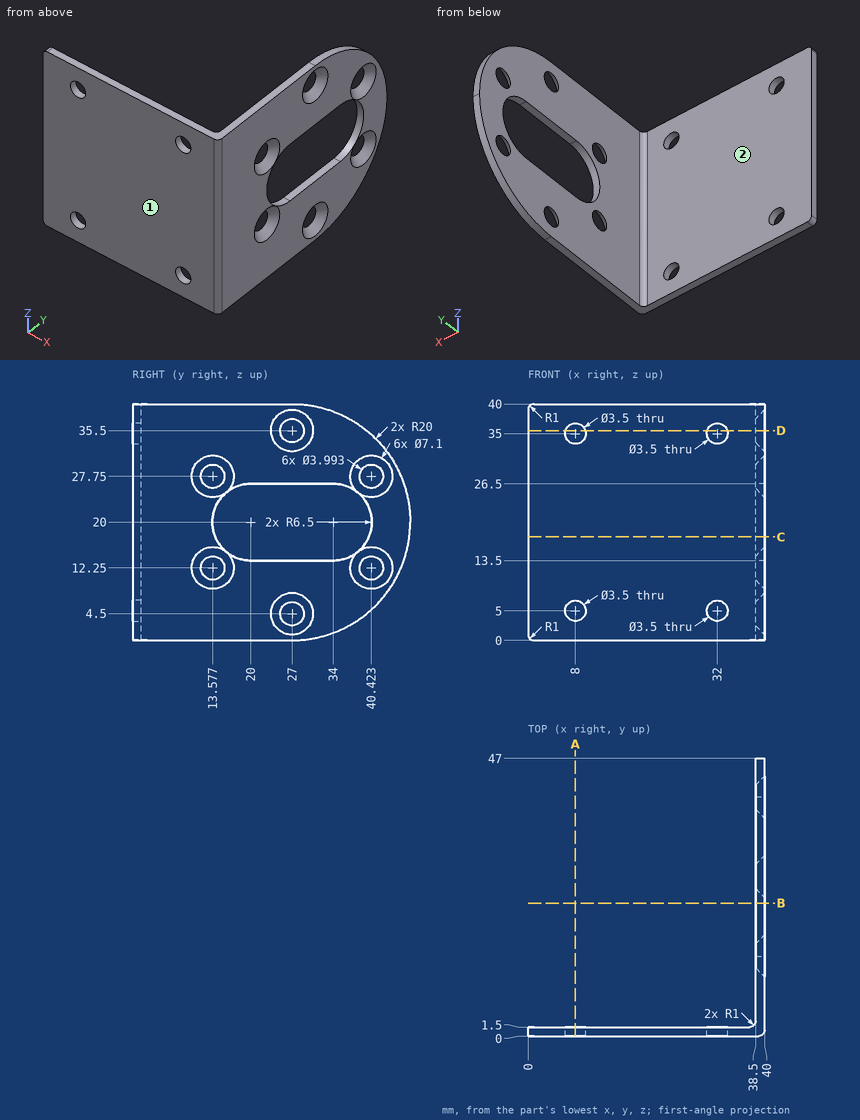
Check sheet for the drawn part. Datum: minimum x, y, z corner. Units: mm. A direction names the side the tool comes from. Give positions to 0.01 mm unless a question says otherwise; leave off trailing zeros. Write each loop counter-clockwise with the first axis right and the second up, starting at its lowest first coordinate (ties: lowest second). Pieces come first, ordered by that corner, then holes. Notation, with made-up numbers: M -31,41 L -6,41 A30 cw -6,64 Z; hole C 39,19.25 d11. An arc over 180 degrees is marked long. One line per question, with ' | ' between items.
1) Section check C-C on z = 17.5. Enter the section's corners in (x, y).
Result:
outline: M 0,0 L 39,0 A1 ccw 40,1 L 40,14 L 38.5,14 L 38.5,2.5 A1 cw 37.5,1.5 L 0,1.5 Z; M 38.5,40 L 40,40 L 40,46.84 L 38.5,46.84 Z
2) Section check A-A on x = 8. Enter the section's corners in (y, z).
Result:
outline: M 0,0 L 1.5,0 L 1.5,3.25 L 0,3.25 Z; M 0,6.75 L 1.5,6.75 L 1.5,33.25 L 0,33.25 Z; M 0,36.75 L 1.5,36.75 L 1.5,40 L 0,40 Z
3) Set-up check for the marked faces 1 and 2: record each of +Z, -Z, +X, -X, +Y, -Y from which the full face is reachable in a straight line by a thin tool's end or side.
Result:
face 1: +Z, -Z, +X, -X, -Y | face 2: +Z, -Z, -X, +Y
4) Thickness scan on line 1 along Y through (x, z) = (7, 23); line 2 along X through (y, z) = (25.5, 10); line 3 along X through (y, z) = (2, 10) (1 decimal). Record the ranges inside material, lowest first. Write a range as [from, to].
Result:
line 1: y = [0, 1.5] | line 2: x = [38.5, 40] | line 3: x = [38.4, 40]
5) Section check B-B on y = 22.5. Enter the section's corners in (x, z).
Result:
outline: M 38.5,0 L 40,0 L 40,13.5 L 38.5,13.5 Z; M 38.5,26.5 L 40,26.5 L 40,40 L 38.5,40 Z
6) Gauge pin test, flat ends, axial feed: pin 1 Ø19 at (x, z) = (12.5, 17.5) entering from +Y; pin 2 Ø6 at (y, z) = (6.5, 24) entering from -X. Record the tip position at first contact, or that the pin passes through.
Result:
pin 1: stops at y = 1.5 | pin 2: stops at x = 38.5
7) Section check D-D on z = 35.5. Enter the section's corners in (x, y).
Result:
outline: M 0,0 L 6.32,0 L 6.32,1.5 L 0,1.5 Z; M 9.68,0 L 30.32,0 L 30.32,1.5 L 9.68,1.5 Z; M 33.68,0 L 39,0 A1 ccw 40,1 L 40,23.45 L 38.5,25 L 38.5,2.5 A1 cw 37.5,1.5 L 33.68,1.5 Z; M 38.5,29 L 40,30.55 L 40,39.64 L 38.5,39.64 Z
